Study the drawing (mm; zero at the part's minimum x, y, z) and answer. A direction names the side the tool comes from. Coordinates: 2 decimals unless noted, no trailing zeros. Order: outer loops, then holes, each group sorted by start corner. A loop starts at its lowest first (then second) coordinate and runs counter-clockwise, first axis right, second up. Notation, with made-up numbers: M 48,60.25 L 83,60.25 A25 ccw 83,82.25 Z; hole C 26.5,36 d9. An arc over 180 degrees is marked long. Use a Markdown table: item, result. Add a question column.
1) Find section A-A on y = 17. Write down the section's boundary in (x, z).
2) Find section B-B on z = 39. Write down the section's boundary in (x, y), plus the area to 3 significant figures.
3) Find section C-C on x = 40. Write down the section's boundary in (y, z), plus the area to 3 significant figures.
4) For the marked faces 1, 2 and 3, determine the directions among +Z, -Z, +X, -X, +Y, -Y from which every point of the face is accessible in a straight line to the end or side of a thin tool.
5) Find section D-D on z = 5. Write down the section's boundary in (x, y), plus the area to 3 significant figures.
6) Find the intervals of material crossed by probe 1 along Y at (x, z) = (35, 29.5) (1 decimal); probe 2 along Y at (x, z) = (34, 10.5); probe 3 along Z at (x, y) = (29, 38), in increasing order. Write a range as [from, to].
7) Each of these flat-tipped pins is pushed along its axis until it touches: pin 1 Ø3 at (x, y) = (12, 55.5) entering from -Z; pin 2 Ø2 at (y, z) = (38, 22) entering from +X; pin 3 Ø1 at (y, z) = (56, 15) entering from -X. Where does it stop, or does it pass through?
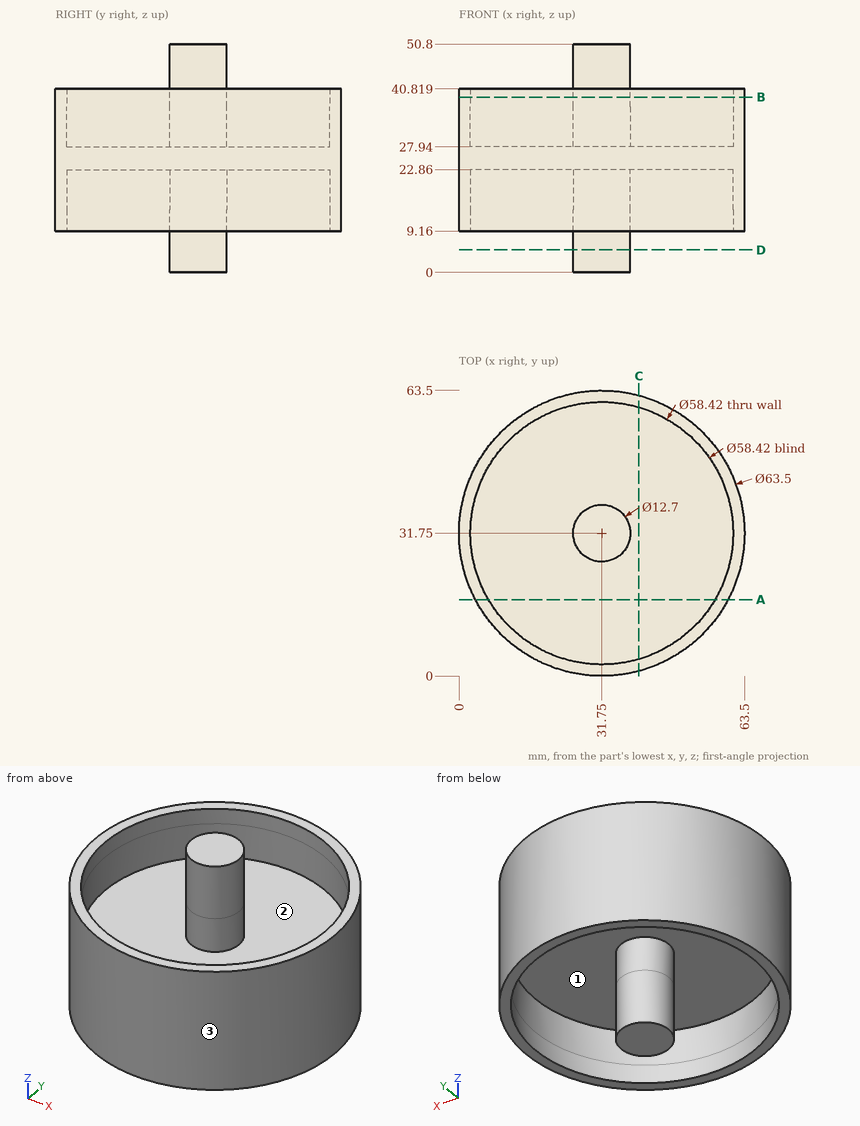
Check result:
| question | item | result |
|---|---|---|
| 1 | outline | M 3.63,9.16 L 6.54,9.16 L 6.54,22.86 L 56.96,22.86 L 56.96,9.16 L 59.87,9.16 L 59.87,40.82 L 56.96,40.82 L 56.96,27.94 L 6.54,27.94 L 6.54,40.82 L 3.63,40.82 Z |
| 2 | outline | C 31.75,31.75 d63.5; C 31.75,31.75 d12.7; hole C 31.75,31.75 d58.42 |
| 2 | area | 613 mm2 |
| 3 | outline | M 1.09,9.16 L 3.73,9.16 L 3.73,22.86 L 59.77,22.86 L 59.77,9.16 L 62.41,9.16 L 62.41,40.82 L 59.77,40.82 L 59.77,27.94 L 3.73,27.94 L 3.73,40.82 L 1.09,40.82 Z |
| 3 | area | 452 mm2 |
| 4 | face 1 | -Z |
| 4 | face 2 | +Z |
| 4 | face 3 | +Z, -Z |
| 5 | outline | C 31.75,31.75 d12.7 |
| 5 | area | 127 mm2 |
| 6 | probe 1 | y = [0.2, 2.7], [26.3, 37.2], [60.8, 63.3] |
| 6 | probe 2 | y = [0.08, 2.63], [25.81, 37.69], [60.87, 63.42] |
| 6 | probe 3 | z = [22.86, 27.94] |
| 7 | pin 1 | stops at z = 9.16 |
| 7 | pin 2 | stops at x = 63.06 |
| 7 | pin 3 | stops at x = 10.68 |
